Verification items for this drawing (mm, ordinates from the low corner). A direction names the side the tool comes from. Coordinates: 2 decimals unless noted, no trailing zeros. Write each loop counter-clockwise with the first axis right and the second up, starting at its lowest first coordinate (ties: lowest second). Pieces come first, ordered by that corner, then holes. Notation, with made-up numbers: M -4,-14.75 L 20,-14.75 A23 ccw 20,-4.75 Z; hole C 54,51.5 d5. An arc over 180 degrees is marked long. Put each result on its own line as item: value. Start each with the question number.
1) Scan lines: line 1 along Z through (x, y) = (132, 23.5); line 2 along Y through (x, z) = (149.5, 30.5); line 3 along X through (y, z) = (55.5, 25.5). Record each from-to range of solid material in increasing order.
2) Cross-section at B-B on x = 23.3. Record the cut outline in (y, z), plus the area to 3 significant figures.
3) Set-up check for the marked faces 1, 2 and 3: record each of +Z, -Z, +X, -X, +Y, -Y from which the full face is reachable in a straight line by a thin tool's end or side.
4) Gauge pin test, flat ends, axial feed: pin 1 (22 mm diameter, centred on x = 131, z = 17.5, fed in from -Y); pin 2 (4 mm diameter, centred on x = 50.5, y = 33.5, fed in from +Z); pin 3 (12 mm diameter, centred on x = 36.5, y = 37.5, fed in from +Z). Record the tip position at first contact, or that the pin passes through.
5) Cross-section at A-A on z = 24. Record the cut outline in (x, y).
6) Cross-section at C-C on y = 30. Record the cut outline in (x, z), plus the area to 3 significant figures.
7) Cross-section at D-D on y = 21. Record the cut outline in (x, z), plus the area to 3 significant figures.
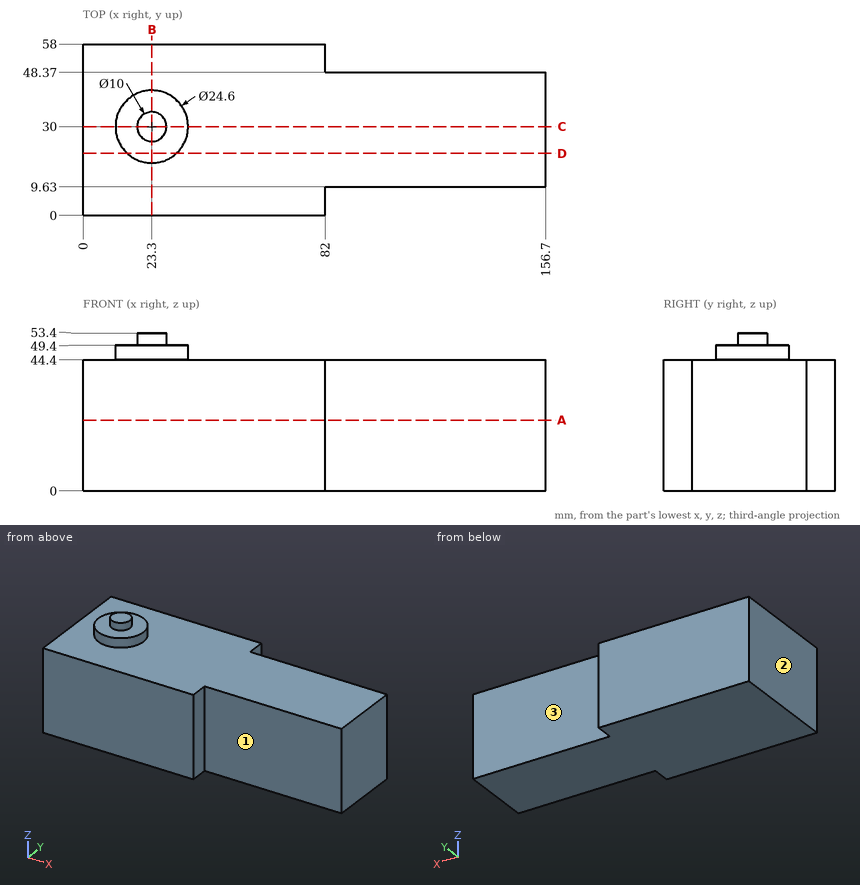
Answer key:
1. line 1: z = 0 to 44.4
1. line 2: y = 9.63 to 48.37
1. line 3: x = 0 to 82
2. outline: M 0,0 L 58,0 L 58,44.4 L 42.3,44.4 L 42.3,49.4 L 35,49.4 L 35,53.4 L 25,53.4 L 25,49.4 L 17.7,49.4 L 17.7,44.4 L 0,44.4 Z
2. area: 2,740 mm²
3. face 1: +Z, -Z, +X, -Y
3. face 2: +Z, -Z, -X, +Y, -Y
3. face 3: +Z, -Z, +X, +Y
4. pin 1: stops at y = 9.63
4. pin 2: stops at z = 44.4
4. pin 3: stops at z = 49.4
5. outline: M 0,0 L 82,0 L 82,9.63 L 156.7,9.63 L 156.7,48.37 L 82,48.37 L 82,58 L 0,58 Z
6. outline: M 0,0 L 156.7,0 L 156.7,44.4 L 35.6,44.4 L 35.6,49.4 L 28.3,49.4 L 28.3,53.4 L 18.3,53.4 L 18.3,49.4 L 11,49.4 L 11,44.4 L 0,44.4 Z
6. area: 7,120 mm²
7. outline: M 0,0 L 156.7,0 L 156.7,44.4 L 31.68,44.4 L 31.68,49.4 L 14.92,49.4 L 14.92,44.4 L 0,44.4 Z
7. area: 7,040 mm²
